Part model, mm, in its own coordinate system. Give positions to 0.01 mm unless a question says otherwise; leave off trailing zeros. Write each loop counter-clockwise with the first axis right and the second up, starting at its lowest first coordinate (ties: lowest second). Pieces come first, ordered by that corner, then holes. Notation, with made-up numbers: M 7,15 L 38,15 A18 ccw 38,36 Z; hole C -30,-29 d9. An arc over 180 degrees is marked long. Use a Markdown table: item, result. Add a question column.
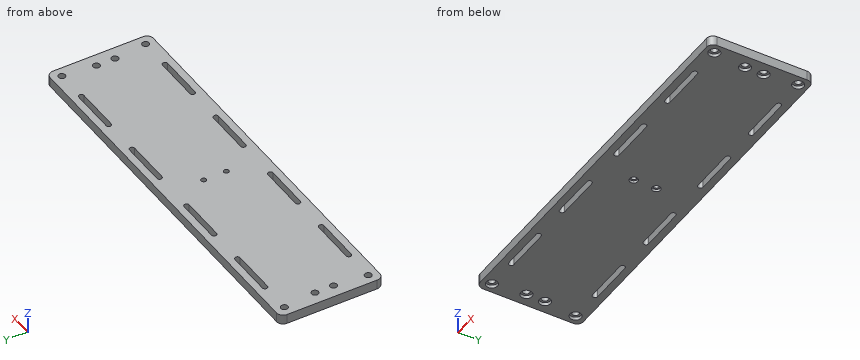
from build123d import *

# Parameters (mm, degrees)
SKETCH1_W                                            = 380.2888
SKETCH1_H                                            = 101.6
BOSS_EXTRUDE1_DEPTH                                  = 9.525
F_10_CLEARANCE_SLOT1_DEPTH                           = 9.525
FILLET1_R                                            = 6.35
CBORE_FOR_1_4_SOCKET_HEAD_CAP_SCREW4_D               = 6.7564
CBORE_FOR_1_4_SOCKET_HEAD_CAP_SCREW4_CBORE_D         = 11.1125
CBORE_FOR_1_4_SOCKET_HEAD_CAP_SCREW4_CBORE_DEPTH     = 3.175
CBORE_FOR_10_SOCKET_HEAD_CAP_SCREW1_D                = 5.1054
CBORE_FOR_10_SOCKET_HEAD_CAP_SCREW1_CBORE_D          = 8.128
CBORE_FOR_10_SOCKET_HEAD_CAP_SCREW1_CBORE_DEPTH      = 2.54
CBORE_FOR_1_4_BINDING_HEAD_MACHINE_SCREW_D           = 6.7564
CBORE_FOR_1_4_BINDING_HEAD_MACHINE_SCREW_DEPTH       = 12.827
CBORE_FOR_1_4_BINDING_HEAD_MACHINE_SCREW_CBORE_D     = 11.1125
CBORE_FOR_1_4_BINDING_HEAD_MACHINE_SCREW_CBORE_DEPTH = 3.175


# Read off the part's stored shape, not the designer's step: #10 Clearance Slot1
with BuildPart() as part:
    # Sketch1 → Boss-Extrude1 (new body)
    with BuildSketch(Plane.XY):
        Rectangle(SKETCH1_W, SKETCH1_H)
    extrude(amount=BOSS_EXTRUDE1_DEPTH)

    # #10 Clearance Slot1 outline → #10 Clearance Slot1 (cut)
    with BuildSketch(Plane.XY):
        with BuildLine():
            Line((-149.0472, 38.7858), (-104.5972, 38.7858))
            ThreePointArc((-104.5972, 38.7858), (-102.108, 41.275), (-104.5972, 43.7642))
            Line((-104.5972, 43.7642), (-149.0472, 43.7642))
            ThreePointArc((-149.0472, 43.7642), (-151.5364, 41.275), (-149.0472, 38.7858))
        make_face()
        with BuildLine():
            ThreePointArc((-22.0472, 38.7858), (-19.558, 41.275), (-22.0472, 43.7642))
            Line((-22.0472, 43.7642), (-66.4972, 43.7642))
            ThreePointArc((-66.4972, 43.7642), (-68.9864, 41.275), (-66.4972, 38.7858))
            Line((-66.4972, 38.7858), (-22.0472, 38.7858))
        make_face()
        with BuildLine():
            ThreePointArc((66.4972, 38.7858), (68.9864, 41.275), (66.4972, 43.7642))
            Line((66.4972, 43.7642), (22.0472, 43.7642))
            ThreePointArc((22.0472, 43.7642), (19.558, 41.275), (22.0472, 38.7858))
            Line((22.0472, 38.7858), (66.4972, 38.7858))
        make_face()
        with BuildLine():
            ThreePointArc((149.0472, 38.7858), (151.5364, 41.275), (149.0472, 43.7642))
            Line((149.0472, 43.7642), (104.5972, 43.7642))
            ThreePointArc((104.5972, 43.7642), (102.108, 41.275), (104.5972, 38.7858))
            Line((104.5972, 38.7858), (149.0472, 38.7858))
        make_face()
        with BuildLine():
            Line((104.5972, -43.7642), (149.0472, -43.7642))
            ThreePointArc((149.0472, -43.7642), (151.5364, -41.275), (149.0472, -38.7858))
            Line((149.0472, -38.7858), (104.5972, -38.7858))
            ThreePointArc((104.5972, -38.7858), (102.108, -41.275), (104.5972, -43.7642))
        make_face()
        with BuildLine():
            ThreePointArc((66.4972, -43.7642), (68.9864, -41.275), (66.4972, -38.7858))
            Line((66.4972, -38.7858), (22.0472, -38.7858))
            ThreePointArc((22.0472, -38.7858), (19.558, -41.275), (22.0472, -43.7642))
            Line((22.0472, -43.7642), (66.4972, -43.7642))
        make_face()
        with BuildLine():
            ThreePointArc((-22.0472, -43.7642), (-19.558, -41.275), (-22.0472, -38.7858))
            Line((-22.0472, -38.7858), (-66.4972, -38.7858))
            ThreePointArc((-66.4972, -38.7858), (-68.9864, -41.275), (-66.4972, -43.7642))
            Line((-66.4972, -43.7642), (-22.0472, -43.7642))
        make_face()
        with BuildLine():
            ThreePointArc((-104.5972, -43.7642), (-102.108, -41.275), (-104.5972, -38.7858))
            Line((-104.5972, -38.7858), (-149.0472, -38.7858))
            ThreePointArc((-149.0472, -38.7858), (-151.5364, -41.275), (-149.0472, -43.7642))
            Line((-149.0472, -43.7642), (-104.5972, -43.7642))
        make_face()
    extrude(amount=F_10_CLEARANCE_SLOT1_DEPTH, mode=Mode.SUBTRACT)

    # Fillet1
    fillet1_edges = [part.edges().sort_by_distance(p)[0] for p in [
        (-190.1444, 50.8, 4.7625),
        (190.1444, 50.8, 4.7625),
        (190.1444, -50.8, 4.7625),
        (-190.1444, -50.8, 4.7625),
    ]]
    fillet(fillet1_edges, radius=FILLET1_R)

    # CBORE for 1/4 Socket Head Cap Screw4 (through all)
    with Locations(Plane(origin=(0, 0, 0), x_dir=(-1, 0, 0), z_dir=(0, 0, -1))):
        with Locations((-177.4444, 9.144), (-177.4444, -9.144), (177.4444, 9.144), (177.4444, -9.144)):
            CounterBoreHole(CBORE_FOR_1_4_SOCKET_HEAD_CAP_SCREW4_D / 2, CBORE_FOR_1_4_SOCKET_HEAD_CAP_SCREW4_CBORE_D / 2, CBORE_FOR_1_4_SOCKET_HEAD_CAP_SCREW4_CBORE_DEPTH)

    # CBORE for #10 Socket Head Cap Screw1 (through all)
    with Locations(Plane(origin=(0, 0, 0), x_dir=(-1, 0, 0), z_dir=(0, 0, -1))):
        with Locations((0, 11.1125), (0, -11.1125)):
            CounterBoreHole(CBORE_FOR_10_SOCKET_HEAD_CAP_SCREW1_D / 2, CBORE_FOR_10_SOCKET_HEAD_CAP_SCREW1_CBORE_D / 2, CBORE_FOR_10_SOCKET_HEAD_CAP_SCREW1_CBORE_DEPTH)

    # CBORE for 1/4 Binding Head Machine Screw1
    with Locations(Plane(origin=(0, 0, 0), x_dir=(-1, 0, 0), z_dir=(0, 0, -1))):
        with Locations((180.6194, 41.275), (180.6194, -41.275), (-180.6194, 41.275), (-180.6194, -41.275)):
            CounterBoreHole(CBORE_FOR_1_4_BINDING_HEAD_MACHINE_SCREW_D / 2, CBORE_FOR_1_4_BINDING_HEAD_MACHINE_SCREW_CBORE_D / 2, CBORE_FOR_1_4_BINDING_HEAD_MACHINE_SCREW_CBORE_DEPTH, depth=CBORE_FOR_1_4_BINDING_HEAD_MACHINE_SCREW_DEPTH)


solid = part.part
1. Cut at B-B (z = 8). Give the number of separate pieces and of enclosed holes in the cut face, then the cut area to 3 significant figures.
2. Cut at A-A (x = 136). Write the cut outline in (y, z) (3 decimals), then the cut area to 3 significant figures.
3. Flat gauge pin, fed straight in: pin 1 (3.5 mm diameter, centred on x = -178.5, y = -10.5, fed in from -Z) (3 decimals). Where does the tip first touch, or does it go through?
4. Drill centre lines: probe 1 along Y at (x, z) = (146, 2.5); probe 2 along X at (y, z) = (-37, 2.5); probe 3 along X at (y, z) = (11, 4.75). Where is each one in solid material? Low to high. Write a range as [from, to].
A:
| question | item | result |
|---|---|---|
| 1 | separate pieces | 1 |
| 1 | enclosed holes | 18 |
| 1 | area | 36,300 mm² |
| 2 | outline | M -50.8,0 L -43.764,0 L -43.764,9.525 L -50.8,9.525 Z; M -38.786,0 L 38.786,0 L 38.786,9.525 L -38.786,9.525 Z; M 43.764,0 L 50.8,0 L 50.8,9.525 L 43.764,9.525 Z |
| 2 | area | 873 mm² |
| 3 | pin 1 | stops at z = 3.175 |
| 4 | probe 1 | y = [-50.8, -43.76], [-38.79, 38.79], [43.76, 50.8] |
| 4 | probe 2 | x = [-190.14, -184.17], [-177.07, 177.07], [184.17, 190.14] |
| 4 | probe 3 | x = [-190.14, -180.27], [-174.62, -2.55], [2.55, 174.62], [180.27, 190.14] |
